Part model, mm, in its own coordinate system. Face numbers are marked on the shaded views. A direction names the side the tool comes from. Round coordinates to 2 decimals unless told otherwise and drop trailing zeros. Write each loop counter-clockwise with the first axis right and the second up, starting at its lowest first coordinate (ties: lowest second). Pieces come first, ordered by that corner, then holes. Notation, with made-up numbers: M 66.5,26.5 L 123.5,26.5 A28 cw 123.5,51.5 Z; hole C 33,50.25 d5. An arc over 180 degrees is marked long. Use a Markdown table: item, result. Add a question column.
1) Wall check: probe 1 along Z at (x, y) = (-0.5, -5.25); probe 2 along Z at (x, y) = (-5, -1.75); probe 3 along Y at (x, z) = (-7.75, 2.25). Give the ranges that are in metal, low to high.
2) Slice it at A-A on x = 4.25. Write the cut outline in (y, z), plus the area to 3 significant figures.
3) Slice it at C-C on y = 2.5. Write the cut outline in (x, z), plus the area to 3 significant figures.
4) Slice it at B-B on z = 2.75. Write the cut outline in (x, y).
5) Slice it at D-D on z = -0.75. Write the cut outline in (x, y), plus the area to 3 significant figures.
6) Drop flat-ended pins along their axis: P1, Ø2, axis at y = 2, z = -1.5, coming from the -X side; P2, Ø1.5, axis at x = 3.5, y = 2.5, coming from the -Z side; P3, Ø7.5, axis at y = -1, z = 6, coming from the -X side. Give the stop position or say it passes through.
7) Two-plate mould, pull along Z, no slides. Class the marked faces 1, 2 and 3: released by +Z, released by -Z, zero draft, split by the parting line, or undercut.
8) Which spindle directions (+Z, -Z, +X, -X, +Y, -Y) get a long thin tool onto all of the face, cutting with end or side? Do the marked faces 4, 5 and 6. Say none if no direction does.
```python
from build123d import *

# Parameters (mm, degrees)
SKETCH1_W           = 17.3
SKETCH1_H           = 15
BOSS_EXTRUDE1_DEPTH = 12.5
CUT_EXTRUDE1_DEPTH  = 15.3
SKETCH3_R           = 1.7
BOSS_EXTRUDE2_DEPTH = 3.5
FILLET1_R           = 0.5


with BuildPart() as part:
    # Sketch1 → Boss-Extrude1 (new body)
    with BuildSketch(Plane.XY):
        Rectangle(SKETCH1_W, SKETCH1_H)
    extrude(amount=BOSS_EXTRUDE1_DEPTH)

    # Sketch2 → Cut-Extrude1 (cut)
    with BuildSketch(Plane.ZY.offset(8.65)):
        Polygon((10.5, 5), (10.5, -5), (8.5, -5), (8.5, -5.7), (5.6, -5.7), (5.6, -5), (3.3, -5), (3.3, -3.5), (2, -3.5), (2, -2), (1, -2), (1, 2), (2, 2), (2, 3.5), (3.3, 3.5), (3.3, 5), (5.6, 5), (5.6, 5.7), (8.5, 5.7), (8.5, 5), align=None)
    extrude(amount=-CUT_EXTRUDE1_DEPTH, mode=Mode.SUBTRACT)

    # Sketch3 → Boss-Extrude2 (add)
    with BuildSketch(Plane(origin=(0, 0, 0), x_dir=(-1, 0, 0), z_dir=(0, 0, -1))):
        with Locations(Location((1.35, 5.8, 0), (0, 0, 180))):
            Circle(SKETCH3_R)
        with Locations(Location((1.35, -5.8, 0), (0, 0, 180))):
            Circle(SKETCH3_R)
    extrude(amount=BOSS_EXTRUDE2_DEPTH)

    # Fillet1
    fillet1_edges = [part.edges().sort_by_distance(p)[0] for p in [
        (-3.05, 5.8, -3.5),
        (-3.05, -5.8, -3.5),
    ]]
    fillet(fillet1_edges, radius=FILLET1_R)


solid = part.part
```
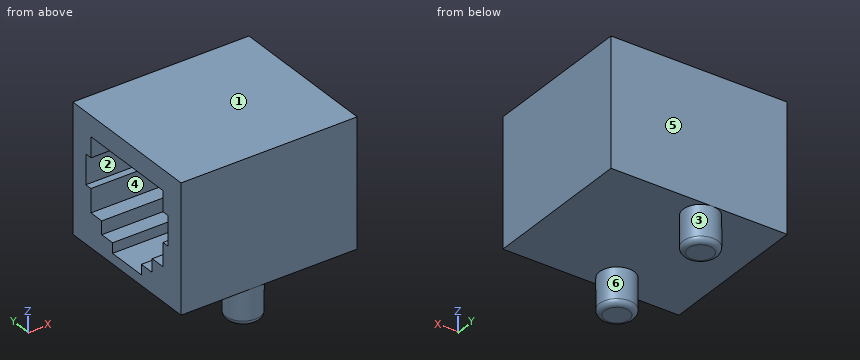
Entries:
| question | item | result |
|---|---|---|
| 1 | probe 1 | z = -3.5 to 5.6, 8.5 to 12.5 |
| 1 | probe 2 | z = 0 to 1, 10.5 to 12.5 |
| 1 | probe 3 | y = -7.5 to -3.5, 3.5 to 7.5 |
| 2 | outline | M -7.5,0 L 7.5,0 L 7.5,12.5 L -7.5,12.5 Z; hole M -5.7,5.6 L -5,5.6 L -5,3.3 L -3.5,3.3 L -3.5,2 L -2,2 L -2,1 L 2,1 L 2,2 L 3.5,2 L 3.5,3.3 L 5,3.3 L 5,5.6 L 5.7,5.6 L 5.7,8.5 L 5,8.5 L 5,10.5 L -5,10.5 L -5,8.5 L -5.7,8.5 Z |
| 2 | area | 98.3 mm^2 |
| 3 | outline | M -8.65,0 L 8.65,0 L 8.65,12.5 L -8.65,12.5 L -8.65,10.5 L 6.65,10.5 L 6.65,2 L -8.65,2 Z |
| 3 | area | 86.2 mm^2 |
| 4 | outline | M -8.65,-7.5 L 8.65,-7.5 L 8.65,7.5 L -8.65,7.5 L -8.65,3.5 L 6.65,3.5 L 6.65,-3.5 L -8.65,-3.5 Z |
| 5 | outline | C -1.35,-5.8 d3.4; C -1.35,5.8 d3.4 |
| 5 | area | 18.2 mm^2 |
| 6 | P1 | passes through |
| 6 | P2 | stops at z = 0 |
| 6 | P3 | stops at x = -8.65 |
| 7 | face 1 | released by +Z |
| 7 | face 2 | undercut |
| 7 | face 3 | zero draft |
| 8 | face 4 | -X |
| 8 | face 5 | +Z, -Z, +X, -X, +Y |
| 8 | face 6 | -Z |
